Check sheet for the modelled part. Datum: model origin and axes. Units: mm. Face numbers are marked on the shaded views. Give positions to 0.01 mm unless a question says otherwise; leave off trailing zeros. Order: outer loops, then holes, each group sorted by start corner. A loop starts at its lowest first (then second) coordinate and runs counter-clockwise, first axis right, second up.
from build123d import *

# Parameters (mm, degrees)
BOSS_EXTRUDE4_DEPTH      = 26.25
BOSS_EXTRUDE4_DEPTH_BACK = 26.25
SKETCH7_W                = 52.75
SKETCH7_H                = 2.5
BOSS_EXTRUDE5_DEPTH      = 27.5
BOSS_EXTRUDE5_DEPTH_BACK = 27.5
SKETCH8_W                = 55
SKETCH8_H                = 2.5
BOSS_EXTRUDE6_DEPTH      = 28.75
BOSS_EXTRUDE6_DEPTH_BACK = 28.75
SKETCH9_W                = 57.5
SKETCH9_H                = 2.5
CUT_EXTRUDE1_DEPTH       = 4
CUT_EXTRUDE1_DEPTH_BACK  = 4.5
SKETCH10_W               = 45.6
SKETCH10_H               = 45.6
SKETCH12_RX              = 7
SKETCH12_RY              = 5
CUT_EXTRUDE2_DEPTH       = 2
CUT_EXTRUDE3_DEPTH       = 29
CUT_EXTRUDE3_DEPTH_BACK  = 42.344588521
SKETCH13_W               = 10
SKETCH13_H               = 3
FILLET4_R                = 1


with BuildPart() as part:
    # Sketch7 → Boss-Extrude4 (new, two sides: drawn at the far end of the back side and taken through both)
    with BuildSketch(Plane.XY.offset(-BOSS_EXTRUDE4_DEPTH_BACK)):
        with Locations((0.125, 1.25)):
            Rectangle(SKETCH7_W, SKETCH7_H)
    extrude(amount=BOSS_EXTRUDE4_DEPTH + BOSS_EXTRUDE4_DEPTH_BACK)

    # Sketch8 → Boss-Extrude5 (add, two sides: drawn at the far end of the back side and taken through both)
    with BuildSketch(Plane.XY.offset(-BOSS_EXTRUDE5_DEPTH_BACK)):
        with Locations((0, 3.75)):
            Rectangle(SKETCH8_W, SKETCH8_H)
    extrude(amount=BOSS_EXTRUDE5_DEPTH + BOSS_EXTRUDE5_DEPTH_BACK)

    # Sketch9 → Boss-Extrude6 (add, two sides: drawn at the far end of the back side and taken through both)
    with BuildSketch(Plane.XY.offset(-BOSS_EXTRUDE6_DEPTH_BACK)):
        with Locations((0, 6.25)):
            Rectangle(SKETCH9_W, SKETCH9_H)
    extrude(amount=BOSS_EXTRUDE6_DEPTH + BOSS_EXTRUDE6_DEPTH_BACK)

    # Sketch10 → Cut-Extrude1 (cut, two sides: drawn at the far end of the back side and taken through both)
    with BuildSketch(Plane(origin=(0, 0, 0), x_dir=(1, 0, 0), z_dir=(0, 1, 0)).offset(-CUT_EXTRUDE1_DEPTH_BACK)):
        Rectangle(SKETCH10_W, SKETCH10_H)
    extrude(amount=CUT_EXTRUDE1_DEPTH + CUT_EXTRUDE1_DEPTH_BACK, mode=Mode.SUBTRACT)

    # Sketch12 → Cut-Extrude2 (cut)
    with BuildSketch(Plane(origin=(0, 7.5, 0), x_dir=(1, 0, 0), z_dir=(0, 1, 0))):
        with Locations((0, 0)):
            Ellipse(SKETCH12_RX, SKETCH12_RY)
    extrude(amount=-CUT_EXTRUDE2_DEPTH, mode=Mode.SUBTRACT)

    # Sketch13 → Cut-Extrude3 (cut, two sides: drawn at the far end of the back side and taken through both)
    with BuildSketch(Plane(origin=(0, 0, 0), x_dir=(1, 0, 0), z_dir=(0, 1, 0)).offset(-CUT_EXTRUDE3_DEPTH_BACK)):
        Rectangle(SKETCH13_W, SKETCH13_H)
    extrude(amount=CUT_EXTRUDE3_DEPTH + CUT_EXTRUDE3_DEPTH_BACK, mode=Mode.SUBTRACT)

    # Fillet4
    fillet4_edges = [part.edges().sort_by_distance(p)[0] for p in [
        (-26.25, 1.25, 26.25),
        (26.5, 1.25, -26.25),
        (0.125, 0, 26.25),
        (26.5, 1.25, 26.25),
        (-27.5, 2.5, 0),
        (-27.5, 3.75, -27.5),
        (27.5, 3.75, -27.5),
        (27.5, 2.5, 0),
        (0, 2.5, -27.5),
        (-27.5, 3.75, 27.5),
        (0, 2.5, 27.5),
        (27.5, 3.75, 27.5),
        (-28.75, 5, 0),
        (-28.75, 6.25, -28.75),
        (28.75, 6.25, -28.75),
        (28.75, 5, 0),
        (0, 5, -28.75),
        (-28.75, 6.25, 28.75),
        (0, 5, 28.75),
        (28.75, 6.25, 28.75),
        (-26.25, 1.25, -26.25),
        (0, 0, -22.8),
        (22.8, 0, 0),
        (0, 0, 22.8),
        (-22.8, 0, 0),
        (26.5, 0, 0),
        (-26.25, 0, 0),
        (0.125, 0, -26.25),
    ]]
    fillet(fillet4_edges, radius=FILLET4_R - 0.0001)  # a hair under: the kernel refuses the full size


solid = part.part
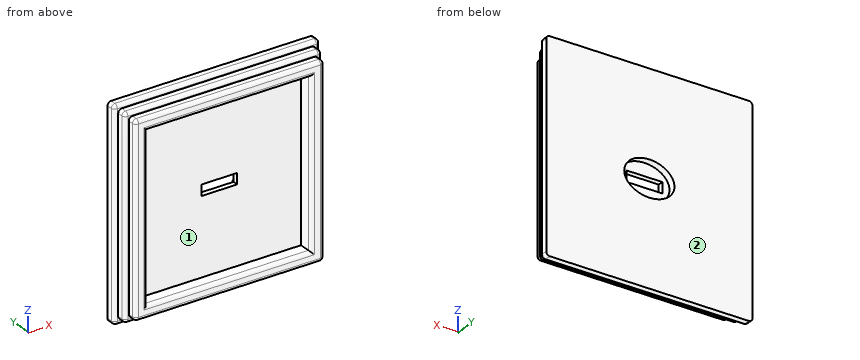
1) Section check A-A, the plane x = -16.5. Record the cut outline in (y, z).
Recorded:
outline: (0, -25.25) arc R1 ccw to (1, -26.25) - (2.5, -26.25) - (2.5, -26.5) arc R1 ccw to (3.5, -27.5) - (5, -27.5) - (5, -27.75) arc R1 ccw to (6, -28.75) - (7.5, -28.75) - (7.5, 28.75) - (6, 28.75) arc R1 ccw to (5, 27.75) - (5, 27.5) - (3.5, 27.5) arc R1 ccw to (2.5, 26.5) - (2.5, 26.25) - (1, 26.25) arc R1 ccw to (0, 25.25) - (0, 23.8) arc R1 ccw to (1, 22.8) - (4, 22.8) - (4, -22.8) - (1, -22.8) arc R1 ccw to (0, -23.8) - close
2) Draft check along X on the marked faces 1 and 2. Enter one of: +X half, -X half, draft (parallel to the pull), parting line (faces both ways), or undercut.
Recorded:
face 1: undercut
face 2: draft
3) Depth check by flat-ended pin: pin 1 Ø1.2 at (y, z) = (4, -8.5) entering from -X; pin 2 Ø0.5 at (x, y) = (1.5, 1.5) entering from -Z; pin 3 Ø0.8 at (x, y) = (0, 5) entering from +Z. Enter the tip coordinate at first touch or a pass-through.
Recorded:
pin 1: stops at x = -27.5
pin 2: stops at z = -26.25
pin 3: stops at z = 28.55
4) Material ranges on L1, parallel to X at y = 2, z = 13; L2, parallel to X at y = 3.75, z = -17, recorded low to high.
Recorded:
L1: x = -26.25 to -22.8, 22.8 to 26.5
L2: x = -27.5 to -22.8, 22.8 to 27.5
